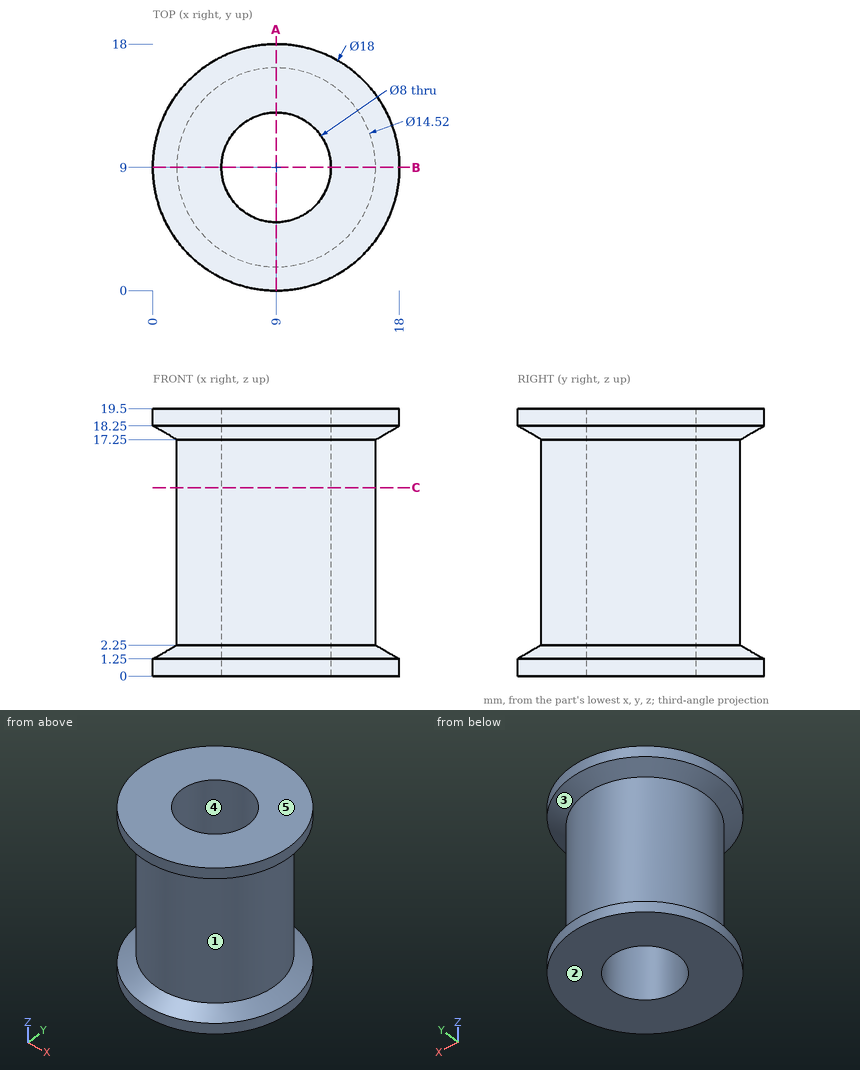
The drawing under review shows one solid part. Ordinate dimensions are in mm from its lowest x, y, z. A direction names the side the tool comes from. Give positions to 0.01 mm unless a question says otherwise; leave off trailing zeros. Write each loop counter-clockwise with the first axis right and the second up, starting at its lowest first coordinate (ties: lowest second). Pieces come first, ordered by that corner, then holes. Notation, with made-up numbers: (-21.5, 84.25) - (-12.5, 84.25) arc R27 cw to (-12.5, 112.25) - close; hole circle Ø10 at (75, 67). An arc over 180 degrees is marked (long way). Answer in a Markdown table with one row per item. Add a question column.
1. Tool access review of the marked faces 1 and 2: name each direction out of +Z, -Z, +X, -X, +Y, -Y from which nothing blocks a thin tool from reaching the whole face with its end or side.
2. Draft analysis for pull direction X (two halves, no side actions). For the marked faces 3, 4 and 5, state which applies: +X half, -X half, draft (parallel to the pull), parting line (faces both ways), or undercut.
3. We need section A-A on x = 9. Write out the cut boundary in (y, z).
4. We need section C-C on z = 13.75. Write out the cut boundary in (x, y).
5. Insertion check: P1, Ø4, axis at x = 12.5, z = 15.5, coming from the +Y side; P2, Ø8, axis at x = 11.5, z = 9, coming from the -Y side; P3, Ø1.5, axis at y = 11, z = 3.5, coming from the +X side. Each pin has a flat end and moves straight along its axis. Give the tip position at first contact, or say it passes through.
6. Wall thickness on line 1 along Y through (x, z) = (9, 8.75); line 2 along Y through (x, z) = (12, 4.5); line 3 along Z through (x, y) = (13.75, 14.75): over which ranges is each line inside the solid? List them lowest first. Write a range as [from, to].
Ans:
| question | item | result |
|---|---|---|
| 1 | face 1 | none |
| 1 | face 2 | -Z, +X, -X, +Y, -Y |
| 2 | face 3 | parting line |
| 2 | face 4 | undercut |
| 2 | face 5 | draft |
| 3 | outline | (0, 0) - (5, 0) - (5, 19.5) - (0, 19.5) - (0, 18.25) - (1.74, 17.25) - (1.74, 2.25) - (0, 1.25) - close; (13, 0) - (18, 0) - (18, 1.25) - (16.26, 2.25) - (16.26, 17.25) - (18, 18.25) - (18, 19.5) - (13, 19.5) - close |
| 4 | outline | circle Ø14.52 at (9, 9); hole circle Ø8 at (9, 9) |
| 5 | P1 | stops at y = 16.1 |
| 5 | P2 | stops at y = 1.74 |
| 5 | P3 | stops at x = 16.15 |
| 6 | line 1 | y = [1.74, 5], [13, 16.26] |
| 6 | line 2 | y = [2.39, 6.35], [11.65, 15.61] |
| 6 | line 3 | z = [0, 2.14], [17.36, 19.5] |
